Check sheet for the drawn part. Datum: minimum x, y, z corner. Units: mm. Coordinates: 2 decimals unless noted, no trailing zeros. Loops run counter-clockwise (first coordinate to the right, second up) from the corner with the lowest first, then second, coordinate; pieces in that order, holes last.
Q1. Sectioned sample at B-B (z = 2.5). Enter the section's corners in (x, y) (1 decimal), then the cut area to 3 significant figures.
Q2. Sectioned sample at D-D (y = 23). Enter the section's corners in (x, z).
Q3. Sectioned sample at C-C (x = 72). Enter the section's corners in (y, z).
Q4. Material ranges on probe 1 along X at (y, z) = (8, 10); probe 2 along Y at (x, z) = (16.5, 18); probe 3 along Y at (x, z) = (24.5, 7.5), recorded low to high.
Q5. Sectioned sample at A-A (z = 10). Enter the section's corners in (x, y) (1 decimal), then the cut area to 3 significant figures.
Q6. Go/stop test with flat-tipped pins: P1, Ø2, axis at x = 52, z = 9, coming from the +Y side; P2, Ø12, axis at x = 37.5, z = 7.5, coming from the +Y side (1 decimal); P3, Ø3.5, axis at x = 50.15, z = 10, coming from the +Y side. Record where each tip stops, or that it passes through.
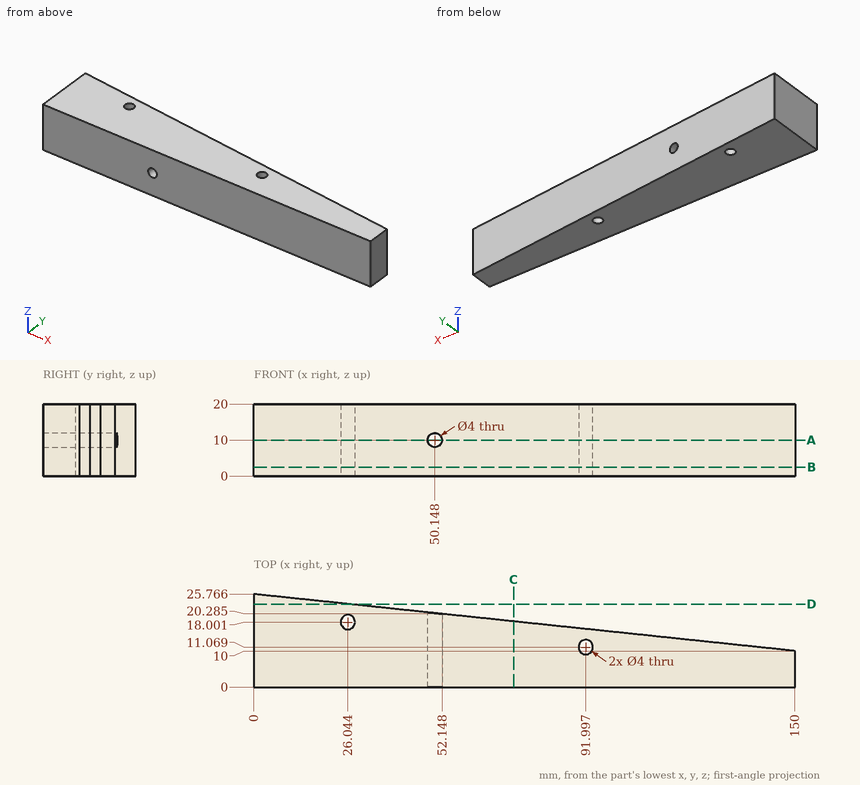
Geometry check:
1. outline: (0, 0) - (150, 0) - (150, 10) - (0, 25.8) - close; hole circle Ø4 at (26, 18); hole circle Ø4 at (92, 11.1)
1. area: 2,660 mm2
2. outline: (0, 0) - (26.31, 0) - (26.31, 20) - (0, 20) - close
3. outline: (0, 0) - (18.2, 0) - (18.2, 20) - (0, 20) - close
4. probe 1: x = 0 to 48.15, 52.15 to 150
4. probe 2: y = 0 to 24.03
4. probe 3: y = 0 to 16.73, 19.27 to 23.19
5. outline: (0, 0) - (48.1, 0) - (48.1, 20.7) - (0, 25.8) - close; (52.1, 0) - (150, 0) - (150, 10) - (52.1, 20.3) - close; hole circle Ø4 at (26, 18); hole circle Ø4 at (92, 11.1)
5. area: 2,580 mm2
6. P1: stops at y = 20.38
6. P2: stops at y = 22.5
6. P3: passes through
